from build123d import *

# Parameters (mm, degrees)
OTHER_M2_OUTLINE_R   = 1
OTHER_M2_DEPTH       = 5
OTHER_M2_2_OUTLINE_R = 1
OTHER_M2_2_DEPTH     = 2
SKETCH_2_R           = 1
EXTRUDE_1_DEPTH      = 4


# Read off the part's stored shape, not the designer's step: M2螺栓镜向
with BuildPart() as part:
    # Other M2 outline → Other M2 (new body)
    with BuildSketch(Plane(origin=(0, 0, 0), x_dir=(1, 0, 0), z_dir=(0, 1, 0))):
        Circle(OTHER_M2_OUTLINE_R)
    extrude(amount=OTHER_M2_DEPTH)

    # Other M2 2 outline → Other M2 2 (add)
    with BuildSketch(Plane(origin=(0, 0, 0), x_dir=(1, 0, 0), z_dir=(0, 1, 0))):
        Polygon((1.634810628, 0.57218372), (0.321879677, 1.701879395), (-1.312930951, 1.129695675), (-1.634810628, -0.57218372), (-0.321879677, -1.701879395), (1.312930951, -1.129695675), align=None)
        Circle(OTHER_M2_2_OUTLINE_R, mode=Mode.SUBTRACT)
    extrude(amount=OTHER_M2_2_DEPTH)

    # 草图2 → 凸台-拉伸1 (add)
    with BuildSketch(Plane(origin=(0, 5, 0), x_dir=(1, 0, 0), z_dir=(0, 1, 0))):
        with Locations(Location((0, 0, 0), (0, 0, 270))):
            Circle(SKETCH_2_R)
    extrude(amount=EXTRUDE_1_DEPTH)


solid = part.part
Model file for the job. Use its own axes, mm. A direction names the side the tool comes from. Round coordinates to 2 decimals unless told otherwise and drop trailing zeros. Loops run counter-clockwise (first coordinate to the right, second up) from the corner with the lowest first, then second, coordinate; pieces in that order, holes last.
1. Band-saw the part on B-B, the plane z = 0.85. List the corners of the cut face in (x, y), and give its area (3 significant figures).
Check values:
outline: (-1.31, 0) - (1.37, 0) - (1.37, 2) - (0.53, 2) - (0.53, 9) - (-0.53, 9) - (-0.53, 2) - (-1.31, 2) - close
area: 12.7 mm2
2. Band-saw the part on D-D, the plane z = -1.35. List the corners of the cut face in (x, y).
Check values:
outline: (-0.68, 0) - (0.73, 0) - (0.73, 2) - (-0.68, 2) - close
3. Band-saw the part on C-C, the plane y = 7. List the corners of the cut face in (x, z).
Check values:
outline: circle Ø2 at (0, 0)
4. Band-saw the part on A-A, the plane x = 0. List the corners of the cut face in (y, z).
Check values:
outline: (0, -1.59) - (2, -1.59) - (2, -1) - (9, -1) - (9, 1) - (2, 1) - (2, 1.59) - (0, 1.59) - close
5. Tool access for faces 1 (the flat face through (-0.988, 0.986, 1.129)), 2 (the cylindrical face through (0, 5, 1)): list every direction of +Z, -Z, +X, -X, +Y, -Y with a clear straight run to the whole face (end or side of a thin tool).
Check values:
face 1: +Z, -X, +Y, -Y
face 2: +Y
6. Wall check: probe 1 along X at (y, z) = (5, 0.05); probe 2 along Y at (x, z) = (-1.25, -1.05); probe 3 along X at (y, z) = (3.25, 0.45). Give the ranges that are in metal, low to high.
Check values:
probe 1: x = -1 to 1
probe 2: y = 0 to 2
probe 3: x = -0.89 to 0.89
